Geometry check sheet. Reference: the model listing, model coordinates, mm. Face numbers are marked on the shaded views. A direction names the side the tool comes from. Coordinates: 2 decimals unless noted, no trailing zeros. Loops run counter-clockwise (first coordinate to the right, second up) from the corner with the lowest first, then second, coordinate; pieces in that order, holes last. Notation, with made-up numbers: (76, 11.5) - (120, 11.5) arc R6 cw to (120, 15.5) - close; hole circle Ø7 at (65.25, 66). An arc over 180 degrees is marked (long way). Write each question's results on one line, items separated by ' | '. Start each with the question number.
(1) Access from +Z, -Z, +X, -X, +Y, -Y to the whole of each face (thin tool, end or side, straight path). Record for the marked faces 1, 2, 3 and 4.
(2) Sectioned sample at C-C (z = 3). Enter the section's corners in (x, y).
(3) Go/stop test with flat-tipped pins: pin 1 Ø2 at (y, z) = (19, -2.5) entering from -X; pin 2 Ø4 at (x, y) = (19.5, -7) entering from -Z; pin 3 Ø3 at (x, z) = (-9, -3) entering from +Y; pin 4 Ø4.5 at (x, y) = (13.5, 15) entering from -Z. Record where each tip stops, or that it passes through.
(4) Sectioned sample at D-D (y = 10.5). Enter the section's corners in (x, z).
(5) Material ranges on probe 1 along Y at (x, z) = (0, 4); probe 2 along X at (y, z) = (-11, 1.5); probe 3 along Z at (x, y) = (3, 21.5), recorded low to high.
(6) Sectioned sample at B-B (y = -7). Enter the section's corners in (x, z).
(7) Mould release check, pull along Y, two halves, no side actions. Record for the marked faces 5, 6, 7 and 8: pulls with the +Y half, pulls with the -Y half, needs draft (parallel to the pull), parting line crosses it, or undercut.
(8) Sectioned sample at A-A (x = 0). Enter the section's corners in (y, z), plus the area to 3 significant figures.
from build123d import *

# Parameters (mm, degrees)
CROQUIS1_R                 = 23.75
SALIENTE_EXTRUIR1_DEPTH    = 6
CROQUIS4_R                 = 22.25
CORTAR_EXTRUIR1_DEPTH      = 1
CROQUIS5_R                 = 19.75
CORTAR_EXTRUIR2_DEPTH      = 2
CORTAR_EXTRUIR2_DEPTH_BACK = 6
CROQUIS6_R                 = 22.25
SALIENTE_EXTRUIR2_DEPTH    = 5
CROQUIS7_R                 = 19.75
CORTAR_EXTRUIR3_DEPTH      = 2.5
REDONDEO1_R                = 1
CORTAR_EXTRUIR4_DEPTH      = 2.5
CORTAR_EXTRUIR5_DEPTH      = 2.5
MATRIZC1_COUNT             = 7
REDONDEO2_R                = 1
REDONDEO3_R                = 1
CROQUIS10_R                = 12.25
CORTAR_EXTRUIR6_DEPTH      = 1.0000001
CORTAR_EXTRUIR6_DEPTH_BACK = 11


with BuildPart() as part:
    # Croquis1 → Saliente-Extruir1 (new body)
    with BuildSketch(Plane.XY):
        Circle(CROQUIS1_R)
    extrude(amount=SALIENTE_EXTRUIR1_DEPTH)

    # Croquis4 → Cortar-Extruir1 (cut)
    with BuildSketch(Plane(origin=(0, 0, 0), x_dir=(-1, 0, 0), z_dir=(0, 0, -1))):
        Circle(CROQUIS4_R)
    extrude(amount=-CORTAR_EXTRUIR1_DEPTH, mode=Mode.SUBTRACT)

    # Croquis5 → Cortar-Extruir2 (cut, two sides)
    with BuildSketch(Plane(origin=(0, 0, 1), x_dir=(-1, 0, 0), z_dir=(0, 0, -1))) as cortar_extruir2_sk:
        Circle(CROQUIS5_R)
    extrude(amount=CORTAR_EXTRUIR2_DEPTH, mode=Mode.SUBTRACT)
    extrude(cortar_extruir2_sk.sketch, amount=-CORTAR_EXTRUIR2_DEPTH_BACK, mode=Mode.SUBTRACT)

    # Croquis6 → Saliente-Extruir2 (add)
    with BuildSketch(Plane(origin=(0, 0, 1), x_dir=(-1, 0, 0), z_dir=(0, 0, -1))):
        Circle(CROQUIS6_R)
    extrude(amount=SALIENTE_EXTRUIR2_DEPTH)

    # Croquis7 → Cortar-Extruir3 (cut)
    with BuildSketch(Plane.XY.offset(1)):
        Circle(CROQUIS7_R)
    extrude(amount=-CORTAR_EXTRUIR3_DEPTH, mode=Mode.SUBTRACT)

    # Redondeo1
    redondeo1_edges = [part.edges().sort_by_distance(p)[0] for p in [
        (-19.75, 0, -1.5),
    ]]
    fillet(redondeo1_edges, radius=REDONDEO1_R)

    # Croquis8 → Cortar-Extruir4 (cut)
    with BuildSketch(Plane(origin=(0, 0, -4), x_dir=(-1, 0, 0), z_dir=(0, 0, -1))):
        with BuildLine():
            Line((-5.5, 21.559510662), (-5.5, 15.821267332))
            ThreePointArc((-5.5, 15.821267332), (0, 16.75), (5.5, 15.821267332))
            Line((5.5, 15.821267332), (5.5, 21.559510662))
            ThreePointArc((5.5, 21.559510662), (0, 22.25), (-5.5, 21.559510662))
        make_face()
    cortar_extruir4 = extrude(amount=-CORTAR_EXTRUIR4_DEPTH, mode=Mode.SUBTRACT)

    # Croquis9 → Cortar-Extruir5 (cut)
    with BuildSketch(Plane(origin=(0, 0, -1.5), x_dir=(-1, 0, 0), z_dir=(0, 0, -1))):
        with BuildLine():
            Line((5.5, 17.92519177), (5.5, 21.559510662))
            ThreePointArc((5.5, 21.559510662), (0, 22.25), (-5.5, 21.559510662))
            Line((-5.5, 21.559510662), (-5.5, 17.92519177))
            ThreePointArc((-5.5, 17.92519177), (0, 18.75), (5.5, 17.92519177))
        make_face()
    cortar_extruir5 = extrude(amount=-CORTAR_EXTRUIR5_DEPTH, mode=Mode.SUBTRACT)

    # MatrizC1: Cortar-Extruir4, Cortar-Extruir5 ×7 about axis
    matrizc1_axis = Axis((0, 0, 0), (0, 0, 1))
    for i in range(1, MATRIZC1_COUNT):
        add(cortar_extruir4.rotate(matrizc1_axis, i * 360 / MATRIZC1_COUNT), mode=Mode.SUBTRACT)
        add(cortar_extruir5.rotate(matrizc1_axis, i * 360 / MATRIZC1_COUNT), mode=Mode.SUBTRACT)

    # Redondeo2
    redondeo2_edges = [part.edges().sort_by_distance(p)[0] for p in [
        (-14.200729992, -8.8826667, -2.75),
        (-16.648460265, 1.841540334, -2.75),
        (-1.909261854, -16.640829882, -2.75),
        (-11.819919401, -11.868108752, -2.75),
        (11.819919401, -11.868108752, -2.75),
        (1.909261854, -16.640829882, -2.75),
        (16.648460265, 1.841540334, -2.75),
        (14.200729992, -8.8826667, -2.75),
        (8.940370983, 14.164471988, -2.75),
        (15.798758803, 5.564325681, -2.75),
        (-5.5, 15.821267332, -2.75),
        (5.5, 15.821267332, -2.75),
        (-15.798758803, 5.564325681, -2.75),
        (-8.940370983, 14.164471988, -2.75),
    ]]
    fillet(redondeo2_edges, radius=REDONDEO2_R)

    # Redondeo3
    redondeo3_edges = [part.edges().sort_by_distance(p)[0] for p in [
        (9.653913195, 20.046557311, -4),
        (21.692146046, 4.951090781, -4),
        (17.395750485, -13.872648091, -4),
        (0, -22.25, -4),
        (-17.395750485, -13.872648091, -4),
        (-21.692146046, 4.951090781, -4),
        (-9.653913195, 20.046557311, -4),
    ]]
    fillet(redondeo3_edges, radius=REDONDEO3_R)

    # Croquis10 → Cortar-Extruir6 (cut, two sides)
    with BuildSketch(Plane(origin=(0, 0, -4), x_dir=(-1, 0, 0), z_dir=(0, 0, -1))) as cortar_extruir6_sk:
        Circle(CROQUIS10_R)
    extrude(amount=CORTAR_EXTRUIR6_DEPTH, mode=Mode.SUBTRACT)
    extrude(cortar_extruir6_sk.sketch, amount=-CORTAR_EXTRUIR6_DEPTH_BACK, mode=Mode.SUBTRACT)


solid = part.part
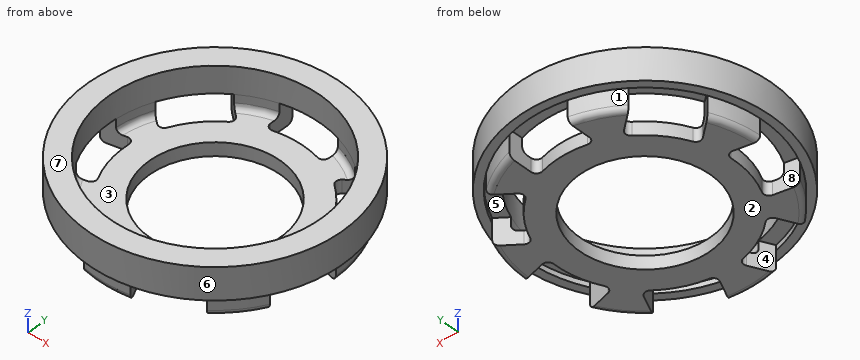
Outcome:
1) face 1: -Z, -X, +Y | face 2: -Z, +X, -X, +Y, -Y | face 3: +Z | face 4: -Z
2) outline: circle Ø47.5 at (0, 0); hole circle Ø39.5 at (0, 0)
3) pin 1: stops at x = -13.08 | pin 2: stops at z = 0 | pin 3: stops at y = 20.95 | pin 4: stops at z = -4
4) outline: (-21.3, 0) - (-19.62, 0) - (-19.62, 1) - (-16.73, 1) - (-16.73, 6) - (-21.3, 6) - close; (-13.05, -4) - (-6.31, -4) - (-6.31, -1.5) - (-13.05, -1.5) - close; (6.31, -4) - (13.05, -4) - (13.05, -1.5) - (6.31, -1.5) - close; (16.73, 1) - (19.62, 1) - (19.62, 0) - (21.3, 0) - (21.3, 6) - (16.73, 6) - close
5) probe 1: y = -23.75 to -19.75, 19.75 to 23.75 | probe 2: x = -21.05 to -16.4, 16.4 to 21.05 | probe 3: z = 1 to 6
6) outline: (-22.69, 0) - (-21.12, 0) - (-21.12, 1) - (-18.47, 1) - (-18.47, 6) - (-22.69, 6) - close; (-15.22, -4) - (-10.05, -4) - (-10.05, -1.5) - (-15.22, -1.5) - close; (10.05, -4) - (15.22, -4) - (15.22, -1.5) - (10.05, -1.5) - close; (18.47, 1) - (21.12, 1) - (21.12, 0) - (22.69, 0) - (22.69, 6) - (18.47, 6) - close
7) face 5: undercut | face 6: parting line crosses it | face 7: needs draft | face 8: undercut
8) outline: (-23.75, 0) - (-22.25, 0) - (-22.25, -3) arc R1 ccw to (-21.25, -4) - (-12.25, -4) - (-12.25, -1.5) - (-18.75, -1.5) arc R1 cw to (-19.75, -0.5) - (-19.75, 6) - (-23.75, 6) - close; (12.25, -4) - (16.75, -4) - (16.75, -1.5) - (12.25, -1.5) - close; (19.75, 1) - (22.25, 1) - (22.25, 0) - (23.75, 0) - (23.75, 6) - (19.75, 6) - close | area: 85.5 mm2
